from build123d import *

# Parameters (mm, degrees)
BOSS_EXTRUDE1_DEPTH = 5
CHAMFER1_SIZE       = 2
SKETCH4_W           = 12
SKETCH4_H           = 3
BOSS_EXTRUDE2_DEPTH = 11.35
BOSS_EXTRUDE3_DEPTH = 3
BOSS_EXTRUDE4_DEPTH = 11.35
CHAMFER2_START      = 116.672618896
CHAMFER2_OUTLINE_W  = 5
CHAMFER2_OUTLINE_H  = 4.65
CHAMFER2_DEPTH      = 2.327381104
CUT_EXTRUDE2_DEPTH  = 2


with BuildPart() as part:
    # Sketch2 → Boss-Extrude1 (new body)
    with BuildSketch(Plane.XY):
        Polygon((-45, 122), (-45, 0.197559457), (-24, -13.44), (24, -13.44), (45, 0.197559457), (45, 122), align=None)
    extrude(amount=BOSS_EXTRUDE1_DEPTH)

    # Chamfer1
    chamfer1_edges = [part.edges().sort_by_distance(p)[0] for p in [
        (45, 122, 2.5),
        (-45, 122, 2.5),
    ]]
    chamfer(chamfer1_edges, length=CHAMFER1_SIZE)

    # Sketch4 → Boss-Extrude2 (add)
    with BuildSketch(Plane.XY.offset(5)):
        Polygon((-45, 120), (-43, 122), (-33, 122), (-33, 119), (-41.757359313, 119), (-42, 118.757359313), (-45, 118.757359313), align=None)
        with Locations((-39, 17.257359313)):
            Rectangle(SKETCH4_W, SKETCH4_H)
        Polygon((0, 122), (30, 122), (30, 108), (27, 108), (27, 119), (0, 119), align=None)
        Polygon((0, 15.757359313), (30, 15.757359313), (30, 29.757359313), (27, 29.757359313), (27, 18.757359313), (0, 18.757359313), align=None)
    extrude(amount=BOSS_EXTRUDE2_DEPTH)

    # Sketch5 → Boss-Extrude3 (add)
    with BuildSketch(Plane.XY.offset(16.35)):
        Polygon((45, 15.757359313), (-45, 15.757359313), (-45, 120), (-43, 122), (45, 122), align=None)
    extrude(amount=BOSS_EXTRUDE3_DEPTH)

    # Sketch6 → Boss-Extrude4 (add)
    with BuildSketch(Plane.XY.offset(5)):
        Polygon((38, 122), (43, 122), (45, 120), (45, 115), (42, 115), (42, 118.757359313), (41.757359313, 119), (38, 119), align=None)
        Polygon((45, 15.757359313), (39, 15.757359313), (39, 18.757359313), (42, 18.757359313), (42, 21.757359313), (45, 21.757359313), align=None)
    extrude(amount=BOSS_EXTRUDE4_DEPTH)

    # Chamfer2: read off the stored shape, not the designer's step
    # Chamfer2 outline → Chamfer2 (cut)
    with BuildSketch(Plane(origin=(0, 0, 0), x_dir=(0.70710678118655, -0.707106781186545, 0), z_dir=(0.707106781186545, 0.70710678118655, 0)).offset(CHAMFER2_START)):
        with Locations((-54.5, -18.675)):
            Rectangle(CHAMFER2_OUTLINE_W, CHAMFER2_OUTLINE_H)
    extrude(amount=CHAMFER2_DEPTH, mode=Mode.SUBTRACT)

    # Sketch8 → Cut-Extrude2 (cut)
    with BuildSketch(Plane.XY.offset(19.35)):
        Polygon((-45, 15.757359313), (-37, 15.757359313), (-37, 122), (-43, 122), (-45, 120), align=None)
    extrude(amount=-CUT_EXTRUDE2_DEPTH, mode=Mode.SUBTRACT)


solid = part.part
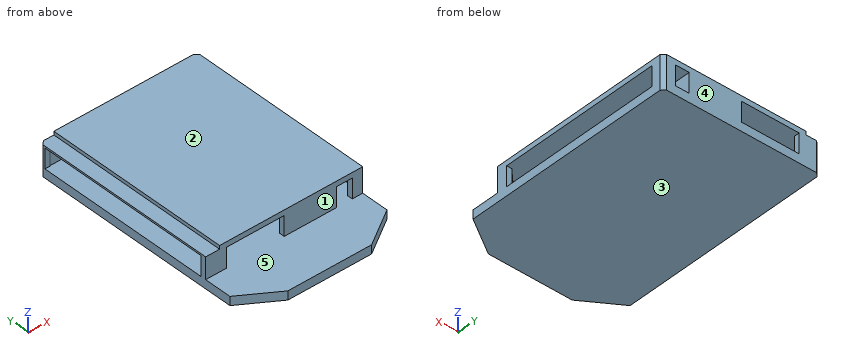
Geometry check sheet. Reference: the model listing, model coordinates, mm. Face numbers are marked on the shaded views. A direction names the side the tool comes from. Round coordinates to 2 decimals unless told otherwise and drop trailing zeros. Order: outer loops, then holes, each group sorted by start corner. A loop starts at its lowest first (then second) coordinate and runs counter-clockwise, first axis right, second up. Notation, with made-up numbers: (-35.75, -15.5) - (-8.75, -15.5) arc R22 ccw to (-8.75, 7.5) - close; hole circle Ø1 at (40.5, 28.25). An arc over 180 degrees is marked (long way). One line per question, with ' | ' between items. Start each with the question number.
(1) Sectioned sample at C-C on z = 2. Record the cut outline in (x, y), and give its area (3 significant figures).
(2) Sectioned sample at A-A on x = -7. Record the cut outline in (y, z), and give its area (3 significant figures).
(3) Access from +Z, -Z, +X, -X, +Y, -Y to the whole of each face (thin tool, end or side, straight path). Record for the marked faces 1 and 2.
(4) Sectioned sample at B-B on y = 101. Record the cut outline in (x, z), and give its area (3 significant figures).
(5) Thickness scan on L1, parallel to Y at x = 20.5, z = 14; L2, parallel to Z at x = 10, y = 69; L3, parallel to X at y = 19, z = 12.5. Record the ranges inside material, lowest first. Write a range as [from, to].
(6) Sectioned sample at D-D on x = 3.5. Record the cut outline in (y, z).
(7) Release check for a two-part mould opening along Z. For the marked faces 3, 4 and 5 record: released by +Z, released by -Z, zero draft, split by the parting line, or undercut.
(8) Depth check by flat-ended pin: pin 1 Ø0.9 at (x, z) = (43.5, 11.5) entering from -Y; pin 2 Ø0.9 at (y, z) = (121, 10.5) entering from -X; pin 3 Ø4.5 at (x, z) = (-18, 9) entering from -Y; pin 4 Ø4 at (y, z) = (116.5, 12.5) entering from -X. Enter the tip coordinate at first touch or a pass-through.
Conclusion:
1) outline: (-45, 0.2) - (-24, -13.44) - (24, -13.44) - (45, 0.2) - (45, 120) - (43, 122) - (-43, 122) - (-45, 120) - close | area: 11,900 mm2
2) outline: (-13.44, 0) - (122, 0) - (122, 5) - (-13.44, 5) - close; (15.76, 16.35) - (122, 16.35) - (122, 19.35) - (15.76, 19.35) - close | area: 996 mm2
3) face 1: +Z, +X, -X, -Y | face 2: +Z, +X, -X, +Y, -Y
4) outline: (-45, 0) - (45, 0) - (45, 5) - (-45, 5) - close; (-45, 16.35) - (45, 16.35) - (45, 19.35) - (-37, 19.35) - (-37, 17.35) - (-45, 17.35) - close | area: 704 mm2
5) L1: y = [15.76, 18.76], [119, 122] | L2: z = [0, 5], [16.35, 19.35] | L3: x = [27, 30], [42, 45]
6) outline: (-13.44, 0) - (122, 0) - (122, 19.35) - (15.76, 19.35) - (15.76, 5) - (-13.44, 5) - close; hole (18.76, 5) - (119, 5) - (119, 16.35) - (18.76, 16.35) - close
7) face 3: released by -Z | face 4: zero draft | face 5: undercut
8) pin 1: stops at y = 15.76 | pin 2: stops at x = -44.45 | pin 3: passes through | pin 4: stops at x = 27
